Could you check a few things on this model? Use its own coordinates, in mm. Give positions to 0.01 mm unless a question says otherwise; leave off trailing zeros. Loops run counter-clockwise (first coordinate to the right, second up) from the corner with the lowest first, then second, coordinate; pieces in that order, holes last. Notation, with made-up numbers: M 87,77.25 L 93,77.25 A12 cw 93,83.25 Z; hole C 78,-17.75 d5. An arc over 180 degrees is marked long. Use a Markdown table: item, result. Add a question column.
1) If I drill on line 1 along X through (y, z) = (-0.3, 10.25); line 2 along Z through (x, y) = (6, -0.3); line 3 along Z through (x, y) = (4.25, -2.75), over which ranges is the centre line in solid material (lowest first)? Write a range as [from, to].
2) Suppose I cut it at B-B on z = 11.75. List the corners of the cut face in (x, y) for me.
3) Suppose I cut it at C-C on y = -3. List the corners of the cut face in (x, z) for me (3 decimals), and give its area (3 significant figures).
4) We'd pull the mould along Z, two halves only. Please class faces 1 (the cylindrical face through (3.864, -2.535, 7.711)), 2 (the flat face through (9, -2, 16)), 3 (the flat face through (0, -2, 8)): +Z half, -Z half, draft (parallel to the pull), parting line (faces both ways), or undercut.
5) Suppose I cut it at A-A on x = 12.5. List the corners of the cut face in (y, z) for me.
```python
from build123d import *

# Parameters (mm, degrees)
F0_W     = 17.32
F0_H     = 16
F1_DEPTH = 5
F2_R     = 1.765
F4_DEPTH = 5
F3_R     = 1.765
F5_DEPTH = 5


with BuildPart() as f1:
    # F0 (on Front) → F1 (new body)
    with BuildSketch(Plane.XZ):
        with Locations((8.66, 8)):
            Rectangle(F0_W, F0_H)
    extrude(amount=F1_DEPTH)

    # F2 (on face) → F4 (cut, through all)
    with BuildSketch(Plane.XZ.offset(5)):
        with Locations((12.855, 10.935)):
            Circle(F2_R)
    extrude(amount=-F4_DEPTH, mode=Mode.SUBTRACT)

    # F3 (on face) → F5 (cut, through all)
    with BuildSketch(Plane.XZ.offset(5)):
        with Locations((5.265, 8.785)):
            Circle(F3_R)
    extrude(amount=-F5_DEPTH, mode=Mode.SUBTRACT)


solid = f1.part
```
Answer block:
| question | item | result |
|---|---|---|
| 1 | line 1 | x = [0, 4.28], [6.25, 11.23], [14.48, 17.32] |
| 1 | line 2 | z = [0, 7.18], [10.39, 16] |
| 1 | line 3 | z = [0, 7.34], [10.23, 16] |
| 2 | outline | M 0,-5 L 11.29,-5 L 11.29,0 L 0,0 Z; M 14.42,-5 L 17.32,-5 L 17.32,0 L 14.42,0 Z |
| 3 | outline | M 0,0 L 17.32,0 L 17.32,16 L 0,16 Z; hole C 5.265,8.785 d3.53; hole C 12.855,10.935 d3.53 |
| 3 | area | 258 mm^2 |
| 4 | face 1 | undercut |
| 4 | face 2 | +Z half |
| 4 | face 3 | draft |
| 5 | outline | M -5,0 L 0,0 L 0,9.21 L -5,9.21 Z; M -5,12.66 L 0,12.66 L 0,16 L -5,16 Z |
